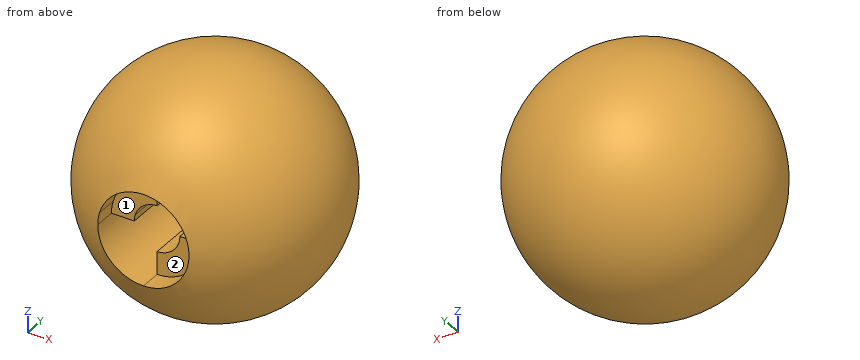
```python
from build123d import *

# Parameters (mm, degrees)
F3_DEPTH = 100
F4_DEPTH = 30
F5_DEPTH = 15
F6_DEPTH = 30


with BuildPart() as f2:
    # F0 (on Top) → F2 (revolve)
    with BuildSketch(Plane.XY):
        with BuildLine():
            Line((40, 0), (-40, 0))
            ThreePointArc((-40, 0), (0, -40), (40, 0))
        make_face()
    revolve(axis=Axis((0, 0, 0), (1, 0, 0)))

    # F1 (on Front) → F3 (cut)
    with BuildSketch(Plane.XZ):
        with BuildLine():
            Line((7.5, 0), (15, 0))
            ThreePointArc((15, 0), (10.606602, 10.606602), (0, 15))
            Line((0, 15), (0, 7.5))
            ThreePointArc((0, 7.5), (-4.522025, 5.983418), (-7.215244, 2.04701))
            Line((-7.215244, 2.04701), (0, 0))
            Line((0, 0), (7.215244, -2.04701))
            ThreePointArc((7.215244, -2.04701), (7.42847, -1.033361), (7.5, 0))
        make_face()
        with BuildLine():
            ThreePointArc((14.430488, -4.094021), (14.85694, -2.066721), (15, 0))
            Line((15, 0), (7.5, 0))
            ThreePointArc((7.5, 0), (7.42847, -1.033361), (7.215244, -2.04701))
            Line((7.215244, -2.04701), (14.430488, -4.094021))
        make_face()
        with BuildLine():
            Line((0, 7.5), (0, 15))
            ThreePointArc((0, 15), (-9.04405, 11.966836), (-14.430488, 4.094021))
            Line((-14.430488, 4.094021), (-7.215244, 2.04701))
            ThreePointArc((-7.215244, 2.04701), (-4.522025, 5.983418), (0, 7.5))
        make_face()
        with BuildLine():
            ThreePointArc((0, -15), (9.04405, -11.966836), (14.430488, -4.094021))
            Line((14.430488, -4.094021), (7.215244, -2.04701))
            ThreePointArc((7.215244, -2.04701), (4.522025, -5.983418), (0, -7.5))
            Line((0, -7.5), (0, -15))
        make_face()
        with BuildLine():
            Line((-7.215244, 2.04701), (-14.430488, 4.094021))
            ThreePointArc((-14.430488, 4.094021), (-14.85694, 2.066721), (-15, 0))
            Line((-15, 0), (-7.5, 0))
            ThreePointArc((-7.5, 0), (-7.42847, 1.033361), (-7.215244, 2.04701))
        make_face()
        with BuildLine():
            ThreePointArc((-15, 0), (-10.606602, -10.606602), (0, -15))
            Line((0, -15), (0, -7.5))
            ThreePointArc((0, -7.5), (4.522025, -5.983418), (7.215244, -2.04701))
            Line((7.215244, -2.04701), (0, 0))
            Line((0, 0), (-7.215244, 2.04701))
            ThreePointArc((-7.215244, 2.04701), (-7.42847, 1.033361), (-7.5, 0))
            Line((-7.5, 0), (-15, 0))
        make_face()
    extrude(amount=F3_DEPTH, mode=Mode.SUBTRACT)

    # F1 (on Front) → F4 (join)
    with BuildSketch(Plane.XZ):
        with BuildLine():
            Line((0, 7.5), (0, 15))
            ThreePointArc((0, 15), (-9.04405, 11.966836), (-14.430488, 4.094021))
            Line((-14.430488, 4.094021), (-7.215244, 2.04701))
            ThreePointArc((-7.215244, 2.04701), (-4.522025, 5.983418), (0, 7.5))
        make_face()
        with BuildLine():
            ThreePointArc((0, -15), (9.04405, -11.966836), (14.430488, -4.094021))
            Line((14.430488, -4.094021), (7.215244, -2.04701))
            ThreePointArc((7.215244, -2.04701), (4.522025, -5.983418), (0, -7.5))
            Line((0, -7.5), (0, -15))
        make_face()
    extrude(amount=F4_DEPTH)

    # F1 (on Front) → F5 (cut)
    with BuildSketch(Plane.XZ):
        with BuildLine():
            Line((0, 7.5), (0, 15))
            ThreePointArc((0, 15), (-9.04405, 11.966836), (-14.430488, 4.094021))
            Line((-14.430488, 4.094021), (-7.215244, 2.04701))
            ThreePointArc((-7.215244, 2.04701), (-4.522025, 5.983418), (0, 7.5))
        make_face()
        with BuildLine():
            ThreePointArc((0, -15), (9.04405, -11.966836), (14.430488, -4.094021))
            Line((14.430488, -4.094021), (7.215244, -2.04701))
            ThreePointArc((7.215244, -2.04701), (4.522025, -5.983418), (0, -7.5))
            Line((0, -7.5), (0, -15))
        make_face()
    extrude(amount=F5_DEPTH, mode=Mode.SUBTRACT)

    # F1 (on Front) → F6 (join)
    with BuildSketch(Plane.XZ):
        with BuildLine():
            Line((-7.215244, 2.04701), (-14.430488, 4.094021))
            ThreePointArc((-14.430488, 4.094021), (-14.85694, 2.066721), (-15, 0))
            Line((-15, 0), (-7.5, 0))
            ThreePointArc((-7.5, 0), (-7.42847, 1.033361), (-7.215244, 2.04701))
        make_face()
        with BuildLine():
            ThreePointArc((14.430488, -4.094021), (14.85694, -2.066721), (15, 0))
            Line((15, 0), (7.5, 0))
            ThreePointArc((7.5, 0), (7.42847, -1.033361), (7.215244, -2.04701))
            Line((7.215244, -2.04701), (14.430488, -4.094021))
        make_face()
    extrude(amount=F6_DEPTH)


solid = f2.part
```
CAD build for the part. Positions are in the model's coordinates, mm. Face numbers are marked on the shaded views. Coordinates: 2 decimals unless noted, no trailing zeros. Order: outer loops, then holes, each group sorted by start corner. A loop starts at its lowest first (then second) coordinate and runs counter-clockwise, first axis right, second up. Notation, with made-up numbers: (5, 9.25) - (18, 9.25) arc R15 ccw to (18, 20.25) - close; hole circle Ø4 at (46.5, 50). An arc over 180 degrees is marked (long way). Use a Markdown table: item, result. Add a question column.
(1) Saw through at C-C (z = 12.5). Give the cut face in (x, y), then the cut area to 3 significant figures.
(2) Saw through at D-D (y = 32). Give the cut face in (x, z), then the cut area to 3 significant figures.
(3) Flat gauge pins, fed straight in: pin 1 (10 mm diameter, centred on x = 17, y = 22.5, fed in from +Z); pin 2 (4.5 mm diameter, centred on x = -7.5, z = 5, fed in from -Y); pin 3 (4 mm diameter, centred on x = -12, y = -15.5, fed in from -Z). Where does each tip first touch, or does it go through?
(4) Saw through at B-B (y = -3). Give the cut face in (x, z).
(5) Saw through at A-A (x = -12). Give the cut face in (y, z), then the cut area to 3 significant figures.
(6) Drill centre lines: line 1 along Z through (x, y) = (13.5, -3); line 2 along Z through (x, y) = (-1, -31); line 3 along Z through (x, y) = (-11, -6). Where is each one in solid material? Low to high. Write a range as [from, to].
(7) Pull direction X, two halves, no side cores. Call the marked faces 1 and 2: +X half, -X half, draft (parallel to the pull), parting line (faces both ways), or undercut.
Solved:
| question | item | result |
|---|---|---|
| 1 | outline | (-8.29, -37.08) - (-8.29, -30) - (0, -30) - (0, -15) - (-8.29, -15) - (-8.29, 0) - (8.29, 0) - (8.29, -37.08) arc R38 ccw (long way) to start |
| 1 | area | 4,030 mm² |
| 2 | outline | circle Ø48 at (0, 0) |
| 2 | area | 1,810 mm² |
| 3 | pin 1 | stops at z = 32.58 |
| 3 | pin 2 | stops at y = -30 |
| 3 | pin 3 | stops at z = -35.92 |
| 4 | outline | circle Ø79.77 at (0, 0); hole (-15, 0) arc R15 ccw to (0, -15) arc R15 ccw to (14.43, -4.09) - (7.22, -2.05) arc R7.5 ccw to (7.5, 0) - (15, 0) arc R15 ccw to (0, 15) arc R15 ccw to (-14.43, 4.09) - (-7.22, 2.05) arc R7.5 ccw to (-7.5, 0) - close |
| 5 | outline | (-37.08, -9) arc R38.16 ccw (long way) to (-37.08, 9) - (-30, 9) - (-30, 0) - (0, 0) - (0, -9) - close; hole (-15, 3.4) - (0, 3.4) - (0, 9) - (-15, 9) - close |
| 5 | area | 4,080 mm² |
| 6 | line 1 | z = [-37.53, -6.54], [-3.83, 0], [6.54, 37.53] |
| 6 | line 2 | z = [-25.26, -14.97], [14.97, 25.26] |
| 6 | line 3 | z = [-37.99, -10.2], [0, 3.12], [10.2, 37.99] |
| 7 | face 1 | undercut |
| 7 | face 2 | undercut |
